CAD build for the part. Positions are in the model's coordinates, mm. Face numbers are marked on the shaded views. A direction names the side the tool comes from. Give positions to 0.01 mm unless a question says otherwise; leave off trailing zeros. Order: outer loops, then holes, each group sorted by start corner. A loop starts at its lowest first (then second) coordinate and runs counter-clockwise, first axis right, second up. Notation, with made-up numbers: (-36.75, -21) -> (-0.75, -21) arc R22 cw to (-0.75, 14) -> close; hole circle Ø8 at (83, -22). An arc over 180 degrees is marked (long way). Use one line per item in the form item = value. Start each with the question number.
1) Cut at B-B, the plane z = 27. Give the cut face in (x, y) (3 decimals), and give its area (3 significant figures).
2) Mould opens along X. For the marked faces 3, 4 and 5 say: pulls with the +X half, pulls with the -X half, needs draft (parallel to the pull), parting line crosses it, or undercut.
3) Probe line 1 (Y direction, x = 12.7, z = 16.25); line 2 (Z direction, x = 12.7, y = -4.25); line 3 (Z direction, x = 3.5, y = -45.5). List the from-to ranges inside material, lowest first.
4) Cut at A-A, the plane z = 44.45. Give the cut face in (x, y).
5) Drop flat-ended pins along their axis: P1, Ø1.5, axis at x = 21, z = 25.5, coming from the -Y side; P2, Ø8.5, axis at x = 12.7, z = 69.85, coming from the -Y side; P3, Ø15, axis at x = 17, y = -33, coming from the +Z side; P4, Ø10, axis at x = 20, y = -32, coming from the -Z side. Give the stop position or say it passes through.
6) Tool access for the marked faces 1 and 2: list every direction of +Z, -Z, +X, -X, +Y, -Y with a clear straight run to the whole face (end or side of a thin tool).
7) Cut at D-D, the plane x = 11.5. Give the cut face in (y, z).
8) Cut at C-C, the plane x = 23.25. Give the cut face in (y, z).
from build123d import *

# Parameters (mm, degrees)
F1_DEPTH = 25.4
F2_R     = 9.525
F2_R_2   = 4.9657
F3_DEPTH = 25.4
F4_R     = 3.2639
F5_DEPTH = 25.4


with BuildPart() as f1:
    # F0 (on Right) → F1 (new body)
    with BuildSketch(Plane.YZ):
        Polygon((-50.8, 0), (0, 0), (0, 82.55), (-6.35, 82.55), (-6.35, 6.35), (-50.8, 6.35), align=None)
    extrude(amount=F1_DEPTH)

    # F2 (on face) → F3 (join)
    with BuildSketch(Plane.XY.offset(6.35)):
        with Locations((12.7, -33.3248)):
            Circle(F2_R)
        with Locations((12.7, -33.3248)):
            Circle(F2_R_2, mode=Mode.SUBTRACT)
    extrude(amount=F3_DEPTH)

    # F4 (on face) → F5 (cut)
    with BuildSketch(Plane.XZ.offset(6.35)):
        with Locations((12.7, 69.85)):
            Circle(F4_R)
        with Locations((13.008095, 44.45)):
            Circle(F4_R)
    extrude(amount=-F5_DEPTH, mode=Mode.SUBTRACT)


solid = f1.part
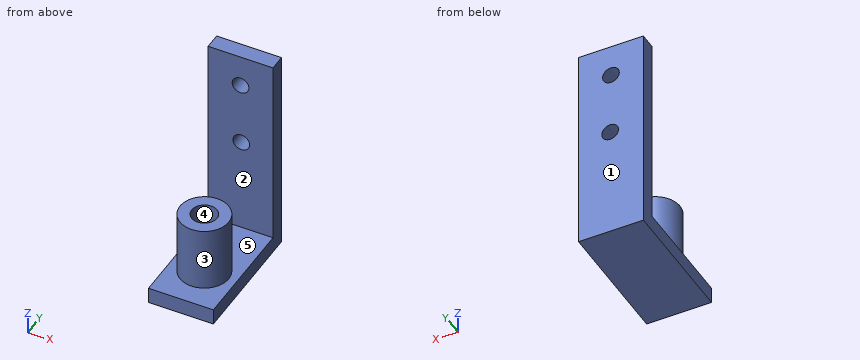
Result:
q1.outline = (0, -6.35) -> (25.4, -6.35) -> (25.4, 0) -> (0, 0) -> close; circle Ø19.05 at (12.7, -33.325); hole circle Ø9.931 at (12.7, -33.325)
q1.area = 369 mm²
q2.face_3 = parting line crosses it
q2.face_4 = undercut
q2.face_5 = needs draft
q3.line_1 = -42.85 to -38.29, -28.36 to -23.8, -6.35 to 0
q3.line_2 = 0 to 41.2, 47.7 to 66.59, 73.11 to 82.55
q3.line_3 = 0 to 6.35
q4.outline = (0, -6.35) -> (9.74, -6.35) -> (9.74, 0) -> (0, 0) -> close; (16.27, -6.35) -> (25.4, -6.35) -> (25.4, 0) -> (16.27, 0) -> close
q5.P1 = -39.13
q5.P2 = -6.35
q5.P3 = 31.75
q5.P4 = 0
q6.face_1 = +Z, -Z, +X, -X, +Y
q6.face_2 = +Z, +X, -X
q7.outline = (-50.8, 0) -> (0, 0) -> (0, 41.56) -> (-6.35, 41.56) -> (-6.35, 6.35) -> (-23.88, 6.35) -> (-23.88, 31.75) -> (-28.51, 31.75) -> (-28.51, 6.35) -> (-38.14, 6.35) -> (-38.14, 31.75) -> (-42.77, 31.75) -> (-42.77, 6.35) -> (-50.8, 6.35) -> close; (-6.35, 47.34) -> (0, 47.34) -> (0, 66.81) -> (-6.35, 66.81) -> close; (-6.35, 72.89) -> (0, 72.89) -> (0, 82.55) -> (-6.35, 82.55) -> close
q8.outline = (-50.8, 0) -> (0, 0) -> (0, 82.55) -> (-6.35, 82.55) -> (-6.35, 6.35) -> (-50.8, 6.35) -> close
